Work out the finished part from the listing and answer in its coordinate system (mm). A direction names the side the tool comes from. Round coordinates to 2 decimals unless told otherwise and drop trailing zeros. Order: outer loops, then holes, each group sorted by start corner. A loop starts at its lowest first (then second) coordinate and runs counter-clockwise, first axis right, second up. Notation, with made-up numbers: M 49,-7 L 73,-7 A11 cw 73,-1 Z; hole C 5,53 d9. An arc over 180 degrees is marked long. Return JSON: item names as keys, results as strings.
from build123d import *

# Parameters (mm, degrees)
F_3_4_16_TAPPED_HOLE1_D            = 17.4625
F_3_4_16_TAPPED_HOLE1_CSINK_D      = 20.32
F_3_4_16_TAPPED_HOLE1_CSINK_ANGLE  = 90
F_9_16_18_TAPPED_HOLE1_D           = 13.09624
F_9_16_18_TAPPED_HOLE1_CSINK_D     = 15.5575
F_9_16_18_TAPPED_HOLE1_CSINK_ANGLE = 90
F_3_8_CLEARANCE_HOLE2_D            = 10.0838
CIRPATTERN1_COUNT                  = 10
SKETCH15_R                         = 3.175
CUT_EXTRUDE1_DEPTH                 = 12.7
F_7_16_20_TAPPED_HOLE1_D           = 9.92124
F_7_16_20_TAPPED_HOLE1_DEPTH       = 14.799358796
F_7_16_20_TAPPED_HOLE1_CSINK_D     = 12.3825
F_7_16_20_TAPPED_HOLE1_CSINK_ANGLE = 90
F_7_16_20_TAPPED_HOLE1_TIP         = 2.980641204
F_7_16_20_TAPPED_HOLE2_D           = 9.92124
F_7_16_20_TAPPED_HOLE2_CSINK_D     = 12.3825
F_7_16_20_TAPPED_HOLE2_CSINK_ANGLE = 90


with BuildPart() as part:
    # Sketch1 → Revolve1 (revolve)
    with BuildSketch(Plane.XY):
        Polygon((0, 0), (-76.2, 0), (-76.2, -25.4), (-58.8899, -25.4), (-58.8899, -22.7076), (-54.8259, -22.7076), (-54.8259, -25.4), (-36.6649, -25.4), (-36.6649, -22.7076), (-32.6009, -22.7076), (-32.6009, -25.4), (-31.0134, -25.4), (-31.0134, -24.765), (-10.9982, -19.812), (0, -13.462186269), align=None)
    revolve(axis=Axis((0, 0, 0), (0, -1, 0)))

    # 3/4-16 Tapped Hole1 (through all)
    with Locations(Plane(origin=(0, 0, 0), x_dir=(1, 0, 0), z_dir=(0, 1, 0))):
        with Locations((0, 0)):
            CounterSinkHole(F_3_4_16_TAPPED_HOLE1_D / 2, F_3_4_16_TAPPED_HOLE1_CSINK_D / 2, counter_sink_angle=F_3_4_16_TAPPED_HOLE1_CSINK_ANGLE)

    # 9/16-18 Tapped Hole1 (through all)
    with Locations(Plane(origin=(0, 0, 0), x_dir=(1, 0, 0), z_dir=(0, 1, 0))):
        with Locations((-44.45, 0), (44.45, 0)):
            CounterSinkHole(F_9_16_18_TAPPED_HOLE1_D / 2, F_9_16_18_TAPPED_HOLE1_CSINK_D / 2, counter_sink_angle=F_9_16_18_TAPPED_HOLE1_CSINK_ANGLE)

    # 3/8 Clearance Hole2 (through all)
    with Locations(Plane(origin=(67.31, 0, 0), x_dir=(0, 0, 1), z_dir=(0, 1, 0))):
        with Locations((0, 0)):
            f_3_8_clearance_hole2 = Hole(F_3_8_CLEARANCE_HOLE2_D / 2)

    # CirPattern1: 3/8 Clearance Hole2 ×10 about axis
    cirpattern1_axis = Axis((0, 0, 0), (0, 1, 0))
    for i in range(1, CIRPATTERN1_COUNT):
        add(f_3_8_clearance_hole2.rotate(cirpattern1_axis, i * 360 / CIRPATTERN1_COUNT), mode=Mode.SUBTRACT)

    # Sketch15 → Cut-Extrude1 (cut, symmetric)
    with BuildSketch(Plane(origin=(0, -2.71901118, -2.71901118), x_dir=(0, 0.7071067811865489, -0.7071067811865462), z_dir=(0, -0.7071067811865462, -0.7071067811865489))):
        with Locations((-27.975262487, 0)):
            Circle(SKETCH15_R)
    extrude(amount=CUT_EXTRUDE1_DEPTH, both=True, mode=Mode.SUBTRACT)

    # 7/16-20 Tapped Hole1
    with Locations(Plane(origin=(0, 0, 26.67), x_dir=(1, 0, 0), z_dir=(0, 1, 0))):
        with Locations((0, 0)):
            CounterSinkHole(F_7_16_20_TAPPED_HOLE1_D / 2, F_7_16_20_TAPPED_HOLE1_CSINK_D / 2, depth=F_7_16_20_TAPPED_HOLE1_DEPTH, counter_sink_angle=F_7_16_20_TAPPED_HOLE1_CSINK_ANGLE)
            with Locations((0, 0, -(F_7_16_20_TAPPED_HOLE1_DEPTH + F_7_16_20_TAPPED_HOLE1_TIP / 2))):  # 118° drill point
                Cone(0, F_7_16_20_TAPPED_HOLE1_D / 2, F_7_16_20_TAPPED_HOLE1_TIP, mode=Mode.SUBTRACT)

    # 7/16-20 Tapped Hole2 (through all)
    with Locations(Plane(origin=(-25.4, 0, -38.1), x_dir=(0, 0, 1), z_dir=(0, 1, 0))):
        with Locations((0, 0)):
            CounterSinkHole(F_7_16_20_TAPPED_HOLE2_D / 2, F_7_16_20_TAPPED_HOLE2_CSINK_D / 2, counter_sink_angle=F_7_16_20_TAPPED_HOLE2_CSINK_ANGLE)


solid = part.part
Item 1: Consider line 1 along Z through (x, y) = (0, -9.5); line 2 along X through (y, z) = (-21.5, -38); line 3 along Z through (x, y) = (-21, -19.5). Determine where each line is inside the solid, lowest interval first. Write a range as [from, to].
Output:
{"line 1": "z = [-76.2, -8.73], [8.73, 21.71], [31.63, 76.2]", "line 2": "x = [-66.05, -59.25], [-49.66, -30.36], [-20.44, 49.66], [59.25, 66.05]", "line 3": "z = [-73.25, -69.05], [-58.98, -40.39], [-35.81, 58.98], [69.05, 73.25]"}
Item 2: Find section A-A (x = 44.45). Determine the outline of the cut face in (y, z).
Output:
{"outline": "M -25.4,-61.89 L 0,-61.89 L 0,-7.78 L -1.23,-6.55 L -25.4,-6.55 L -25.4,-32.09 L -22.71,-32.09 L -22.71,-38.63 L -25.4,-38.63 Z; M -25.4,6.55 L -1.23,6.55 L 0,7.78 L 0,61.89 L -25.4,61.89 L -25.4,38.63 L -22.71,38.63 L -22.71,32.09 L -25.4,32.09 Z"}
Item 3: Each of these flat-tipped pins is pushed along its axis until it touches: pin 1 (11.5 mm diameter, centred on x = -54.45, z = 39.56, fed in from +Y); pin 2 (2 mm diameter, centred on x = 30.5, y = -10, fed in from +Z); pin 3 (11.5 mm diameter, centred on x = 0, z = 26.67, fed in from +Y); pin 4 (10 mm diameter, centred on y = -19, z = 9.5, fed in from +X). Where does it stop, or does it pass through?
Output:
{"pin 1": "stops at y = 0", "pin 2": "stops at z = 70.26", "pin 3": "stops at y = -0.44", "pin 4": "stops at x = 76.07"}
Item 4: Find section B-B (y = -4.5). State how many separate pieces and enclosed holes the cut face has, plus the area to 3 significant figures.
Output:
{"separate pieces": "1", "enclosed holes": "15", "area": "16,800 mm^2"}
Item 5: Find section D-D (z = -48.5). Determine the outline of the cut face in (x, y), plus the area to 3 significant figures.
Output:
{"outline": "M -58.77,-25.4 L -33.4,-25.4 L -33.4,-22.71 L -25.57,-22.71 L -25.57,-25.4 L 25.57,-25.4 L 25.57,-22.71 L 33.4,-22.71 L 33.4,-25.4 L 58.77,-25.4 L 58.77,0 L -58.77,0 Z", "area": "2,940 mm^2"}
Item 6: Which of the six approach directions +Z, -Z, +X, -X, +Y, -Y give full straight-line access (tool end or side, diameter ignored) to faces 1 (the cylindrical face through (51, -13, 0)), 2 (the flat face through (25, -22.708, 22))?
Output:
{"face 1": "+Y, -Y", "face 2": "-Y"}
Item 7: The mould has two halves that part along Y. Classify faces 3 (the flat face through (-39, -22.708, 39)), 4 (the cylindrical face through (-21.63, -12.878, -59.043)), 5 (the cylindrical face through (1, -16.8, 18.5)): pulls with the +Y half, pulls with the -Y half, needs draft (parallel to the pull), parting line crosses it, or undercut.
Output:
{"face 3": "pulls with the -Y half", "face 4": "needs draft", "face 5": "undercut"}
